Read the model definition and answer for the solid it produces. Units are mm, in the model's axes. A direction names the side the tool comes from. Coordinates: 2 decimals unless noted, no trailing zeros. Write each loop counter-clockwise with the first axis right and the second up, starting at its lowest first coordinate (ties: lowest second). Pieces come first, ordered by that corner, then holes. Notation, with made-up numbers: (65, -14.75) -> (87, -14.75) arc R12 ccw to (87, -3.75) -> close; hole circle Ø10 at (10, -32). An arc over 180 degrees is marked (long way). Use CSV: the item, a comma, the result in double quotes. Start each with the question number.
from build123d import *
from build123d.topology import SkipClean

# Parameters (mm, degrees)
BOSS_EXTRUDE1_START     = 3
SKETCH1_W               = 130
SKETCH1_H               = 16
BOSS_EXTRUDE1_DEPTH     = 6
BOSS_EXTRUDE2_START     = 3
SKETCH2_R               = 12
BOSS_EXTRUDE2_DEPTH     = 6
BOSS_EXTRUDE3_START     = 3
SKETCH3_R               = 14
BOSS_EXTRUDE3_DEPTH     = 6
BOSS_EXTRUDE4_START     = 2.5
SKETCH4_R               = 14
BOSS_EXTRUDE4_DEPTH     = 8
CUT_EXTRUDE1_DEPTH      = 146.059470563
CUT_EXTRUDE1_DEPTH_BACK = 146.059470563
SKETCH5_R               = 3.25
CUT_EXTRUDE2_DEPTH      = 146.059470563
CUT_EXTRUDE2_DEPTH_BACK = 146.059470563
SKETCH6_R               = 1.725
CUT_EXTRUDE3_START      = 3
SKETCH7_R               = 2.9
CUT_EXTRUDE3_DEPTH      = 2.2
CUT_EXTRUDE4_START      = 3
SKETCH8_R               = 2.9
CUT_EXTRUDE4_DEPTH      = 2.2
CUT_EXTRUDE5_START      = 3.5
SKETCH9_R               = 11
CUT_EXTRUDE5_DEPTH      = 7
CUT_EXTRUDE6_DEPTH      = 146.059470563
CUT_EXTRUDE6_DEPTH_BACK = 146.059470563
SKETCH10_R              = 8
CUT_EXTRUDE7_START      = 5
SKETCH11_R              = 2
CUT_EXTRUDE7_DEPTH      = 4


with BuildPart() as part:
    # Sketch1 → Boss-Extrude1 (new body)
    with BuildSketch(Plane.XY.offset(BOSS_EXTRUDE1_START)):
        with Locations((65, 0)):
            Rectangle(SKETCH1_W, SKETCH1_H)
    extrude(amount=BOSS_EXTRUDE1_DEPTH)

    # Sketch2 → Boss-Extrude2 (add)
    with BuildSketch(Plane.XY.offset(BOSS_EXTRUDE2_START)):
        Circle(SKETCH2_R)
    extrude(amount=BOSS_EXTRUDE2_DEPTH)

    # Sketch3 → Boss-Extrude3 (add)
    with BuildSketch(Plane.XY.offset(BOSS_EXTRUDE3_START)):
        with Locations((130, 0)):
            Circle(SKETCH3_R)
    extrude(amount=BOSS_EXTRUDE3_DEPTH)

    # Sketch4 → Boss-Extrude4 (add)
    with SkipClean():  # the faces are left unmerged after this step: merging them gives an invalid solid
        with BuildSketch(Plane.XY.offset(BOSS_EXTRUDE4_START)):
            with Locations((130, 0)):
                Circle(SKETCH4_R)
        extrude(amount=BOSS_EXTRUDE4_DEPTH)
    add(part.part.scale(1), mode=Mode.REPLACE)  # the faces are merged on a copy

    # Sketch5 → Cut-Extrude1 (cut, two sides: drawn at the far end of the back side and taken through both)
    with BuildSketch(Plane.XY.offset(-CUT_EXTRUDE1_DEPTH_BACK)):
        Circle(SKETCH5_R)
    extrude(amount=CUT_EXTRUDE1_DEPTH + CUT_EXTRUDE1_DEPTH_BACK, mode=Mode.SUBTRACT)

    # Sketch6 → Cut-Extrude2 (cut, two sides: drawn at the far end of the back side and taken through both)
    with BuildSketch(Plane.XY.offset(-CUT_EXTRUDE2_DEPTH_BACK)):
        with Locations((8, 0)):
            Circle(SKETCH6_R)
        with Locations((20, 0)):
            Circle(SKETCH6_R)
    extrude(amount=CUT_EXTRUDE2_DEPTH + CUT_EXTRUDE2_DEPTH_BACK, mode=Mode.SUBTRACT)

    # Sketch7 → Cut-Extrude3 (cut)
    with BuildSketch(Plane.XY.offset(CUT_EXTRUDE3_START)):
        with Locations((8, 0)):
            Circle(SKETCH7_R)
    extrude(amount=CUT_EXTRUDE3_DEPTH, mode=Mode.SUBTRACT)

    # Sketch8 → Cut-Extrude4 (cut)
    with BuildSketch(Plane.XY.offset(CUT_EXTRUDE4_START)):
        with Locations((20, 0)):
            Circle(SKETCH8_R)
    extrude(amount=CUT_EXTRUDE4_DEPTH, mode=Mode.SUBTRACT)

    # Sketch9 → Cut-Extrude5 (cut)
    with BuildSketch(Plane.XY.offset(CUT_EXTRUDE5_START)):
        with Locations((130, 0)):
            Circle(SKETCH9_R)
    extrude(amount=CUT_EXTRUDE5_DEPTH, mode=Mode.SUBTRACT)

    # Sketch10 → Cut-Extrude6 (cut, two sides: drawn at the far end of the back side and taken through both)
    with BuildSketch(Plane.XY.offset(-CUT_EXTRUDE6_DEPTH_BACK)):
        with Locations((130, 0)):
            Circle(SKETCH10_R)
    extrude(amount=CUT_EXTRUDE6_DEPTH + CUT_EXTRUDE6_DEPTH_BACK, mode=Mode.SUBTRACT)

    # Sketch11 → Cut-Extrude7 (cut)
    with BuildSketch(Plane.XY.offset(CUT_EXTRUDE7_START)):
        with Locations((50, 0)):
            Circle(SKETCH11_R)
        with Locations((90, 0)):
            Circle(SKETCH11_R)
    extrude(amount=CUT_EXTRUDE7_DEPTH, mode=Mode.SUBTRACT)


solid = part.part
1) Each of these flat-tipped pins is pushed along its axis until it touches: pin 1 (1.5 mm diameter, centred on x = 66, z = 7, fed in from +Y); pin 2 (4 mm diameter, centred on x = 7.5, y = 9.5, fed in from +Z); pin 3 (3 mm diameter, centred on x = 8, y = 0, fed in from +Z); pin 4 (3 mm diameter, centred on y = -6.5, z = 4.5, fed in from -X). Where does it stop, or does it pass through?
2) Find the intervals of material crossed by line 1 along X through (y, z) = (-8.75, 7.5); line 2 along Y through (x, z) = (90, 6.5); line 3 along X through (y, z) = (2.5, 5), in increasing order.
3) Section A-A, the plane x = 0 is taken. Give the vertices of the cut face in (y, z), plus the area to 3 significant figures.
4) Section B-B, the plane z = 7.5 is taken. Give the vertices of the cut face in (x, y) (3 decimals), plus the area to 3 significant figures.
5) The mould has two halves that part along Y. Classify faces 1 (the face through (63, -8, 6)), 2 (the face through (52, 0, 3)), 3 (the face through (51.847, -0.766, 6.972)): pulls with the +Y half, pulls with the -Y half, needs draft (parallel to the pull), parting line crosses it, or undercut.
6) Which of the six approach directions +Z, -Z, +X, -X, +Y, -Y give full straight-line access (tool end or side, diameter ignored) to faces 4 (the face through (5.1, 0.1, 4.1)), 5 (the face through (128, -8, 3.5)), 6 (the face through (136.2, -9.3, 10.5))?
7) Section D-D, the plane x = 20 is taken. Give the vertices of the cut face in (y, z) (3 decimals).
8) Section C-C, the plane y = 0 is taken. Count the separate pieces of the cut face and the enclosed holes in it, plus the area to 3 significant figures.
The answers:
1,pin 1,"stops at y = 8"
1,pin 2,"stops at z = 9"
1,pin 3,"passes through"
1,pin 4,"stops at x = -10.91"
2,line 1,"x = -8.21 to 8.21, 119.07 to 123.33, 136.67 to 140.93"
2,line 2,"y = -8 to -2, 2 to 8"
2,line 3,"x = -11.74 to -2.08, 2.08 to 6.53, 9.47 to 18.53, 21.47 to 119.29, 140.71 to 143.77"
3,outline,"(-12, 3) -> (-3.25, 3) -> (-3.25, 9) -> (-12, 9) -> close; (3.25, 3) -> (12, 3) -> (12, 9) -> (3.25, 9) -> close"
3,area,"105 mm^2"
4,outline,"(8.944, -8) -> (118.511, -8) arc R14 ccw (long way) to (118.511, 8) -> (8.944, 8) arc R12 ccw (long way) to start; hole circle Ø6.5 at (0, 0); hole circle Ø3.45 at (8, 0); hole circle Ø3.45 at (20, 0); hole circle Ø4 at (50, 0); hole circle Ø4 at (90, 0); hole circle Ø22 at (130, 0)"
4,area,"2,300 mm^2"
5,face 1,"pulls with the -Y half"
5,face 2,"needs draft"
5,face 3,"undercut"
6,face 4,"-Z"
6,face 5,"+Z"
6,face 6,"+Z, +X, -X, +Y, -Y"
7,outline,"(-8, 3) -> (-2.9, 3) -> (-2.9, 5.2) -> (-1.725, 5.2) -> (-1.725, 9) -> (-8, 9) -> close; (1.725, 5.2) -> (2.9, 5.2) -> (2.9, 3) -> (8, 3) -> (8, 9) -> (1.725, 9) -> close"
8,separate pieces,"5"
8,enclosed holes,"0"
8,area,"699 mm^2"
